For this review, take the finished solid that the model builds, in its own axes (mm). Give positions to 0.01 mm unless a question says otherwise; leave off trailing zeros. Order: outer loops, then holes, each group sorted by start corner. A loop starts at its lowest first (then second) coordinate and runs counter-clockwise, first axis right, second up. Notation, with made-up numbers: M 55,50 L 67,50 A26 ccw 67,67 Z; hole C 86.25,71 d11. An arc over 180 degrees is marked long. Use CSV: the item, a comma, the result in double quotes. Start each with the question number.
(1) Clearance check with flat-ended pins moving along their axes: P1, Ø3, axis at x = 5, z = 441.5, coming from the +Y side; P2, Ø1.9, axis at x = 4.5, y = 42.5, coming from the -Z side. State where each tip first meets the part, or that it passes through.
(2) Consider section A-A (y = 10.5). Write out the cut boundary in (x, z), and give its area (3 significant figures).
(3) Wall thickness on L1, parallel to Z at x = 1.25, y = 43: over which ranges is the line inside the solid? List them lowest first. Write a range as from..to.
Autodesk Inventor part; units mm, degrees
ref_plane "YZ Plane" through (0, 0, 0) normal (1, 0, 0) x (0, 1, 0)
ref_plane "XZ Plane" through (0, 0, 0) normal (0, 1, 0) x (-1, 0, 0)
ref_plane "XY Plane" through (0, 0, 0) normal (0, 0, 1) x (1, 0, 0)
sketch "Sketch1" plane through (0, 0, 0) normal (1, 0, 0) x (0, 1, 0)
  line L0 (-19.05, 443.8029) -> (-19.05, -99.1221)
  line L1 (45.3898, -92.7721) -> (45.3898, 437.4529)
  line L2 (19.9898, 443.8029) -> (19.9898, 437.4529)
  line L3 (19.9898, 437.4529) -> (0, 437.4529)
  line L4 (0, 437.4529) -> (0, 443.8029)
  line L5 (39.0398, 443.8029) -> (39.0398, 437.4529)
  line L6 (39.0398, 437.4529) -> (45.3898, 437.4529)
  line L7 (39.0398, -99.1221) -> (39.0398, -92.7721)
  line L8 (39.0398, -92.7721) -> (45.3898, -92.7721)
  line L9 (0, -99.1221) -> (0, -92.7721)
  line L10 (0, -92.7721) -> (19.9898, -92.7721)
  line L11 (19.9898, -92.7721) -> (19.9898, -99.1221)
  line L12 (39.0398, 443.8029) -> (19.9898, 443.8029)
  line L13 (0, 443.8029) -> (-19.05, 443.8029)
  line L14 (-19.05, -99.1221) -> (0, -99.1221)
  line L15 (19.9898, -99.1221) -> (39.0398, -99.1221)
  point P0 (0, 0)
  dimension "d12" = 6.35
  dimension "d13" = 6.35
  dimension "d14" = 19.05
  dimension "d15" = 19.9898
  dimension "d16" = 6.35
  dimension "d17" = 64.4398
  dimension "d18" = 6.35
  dimension "d19" = 6.35
  dimension "d20" = 19.05
  dimension "d21" = 19.9898
  dimension "d22" = 6.35
  dimension "d23" = 542.925
  dimension "d26" = 6.35
extrude "Extrusion1" add sketch "Sketch1" along normal blind 6.35
properties part number "Front V3"
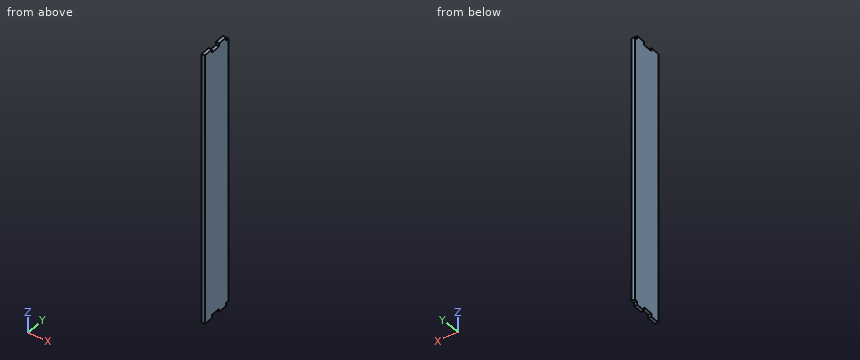
Check result:
1,P1,"stops at y = 39.04"
1,P2,"stops at z = -92.77"
2,outline,"M 0,-92.77 L 6.35,-92.77 L 6.35,437.45 L 0,437.45 Z"
2,area,"3,370 mm^2"
3,L1,"z = -92.77..437.45"
